from build123d import *

# Parameters (mm, degrees)
F0_W      = 42
F0_H      = 27
F1_DEPTH  = 3
F0_H_2    = 3
F2_DEPTH  = 45
F4_D      = 4
F6_D      = 5
F7_R      = 12
F8_DEPTH  = 25
F9_W      = 27
F9_H      = 3
F10_DEPTH = 4
F11_W     = 3
F11_H     = 4
F12_DEPTH = 25
F13_W     = 27
F13_H     = 3
F14_DEPTH = 4
F15_W     = 3
F15_H     = 4
F16_DEPTH = 25


with BuildPart() as f1:
    # F0 (on Top) → F1 (new body)
    with BuildSketch(Plane.XY):
        with Locations((0, 1.5)):
            Rectangle(F0_W, F0_H)
    extrude(amount=F1_DEPTH)

    # F0 (on Top) → F2 (join)
    with BuildSketch(Plane.XY):
        with Locations((0, -13.5)):
            Rectangle(F0_W, F0_H_2)
    extrude(amount=F2_DEPTH)

    # F4 (through all)
    with Locations(Plane.XY.offset(3)):
        with Locations((10, -8.5), (10, 11.5), (-10, 11.5), (-10, -8.5)):
            Hole(F4_D / 2)

    # F6 (through all)
    with Locations(Plane(origin=(0, -12, 0), x_dir=(-1, 0, 0), z_dir=(0, 1, 0))):
        with Locations((-15.5, 39.5), (-15.5, 8.5), (15.5, 8.5), (15.5, 39.5)):
            Hole(F6_D / 2)

    # F7 (on face) → F8 (cut)
    with BuildSketch(Plane(origin=(0, -12, 0), x_dir=(-1, 0, 0), z_dir=(0, 1, 0))):
        with Locations((0, 24)):
            Circle(F7_R)
    extrude(amount=-F8_DEPTH, mode=Mode.SUBTRACT)

    # F9 (on face) → F10 (join)
    with BuildSketch(Plane(origin=(-21, 0, 0), x_dir=(0, -1, 0), z_dir=(-1, 0, 0))):
        with Locations((-1.5, 1.5)):
            Rectangle(F9_W, F9_H)
    extrude(amount=F10_DEPTH)

    # F11 (on face) → F12 (cut)
    with BuildSketch(Plane.XY.offset(3)):
        with Locations((-23.5, 11)):
            Rectangle(F11_W, F11_H)
        with Locations((-23.5, -8)):
            Rectangle(F11_W, F11_H)
    extrude(amount=-F12_DEPTH, mode=Mode.SUBTRACT)

    # F13 (on face) → F14 (join)
    with BuildSketch(Plane.YZ.offset(21)):
        with Locations((1.5, 1.5)):
            Rectangle(F13_W, F13_H)
    extrude(amount=F14_DEPTH)

    # F15 (on face) → F16 (cut)
    with BuildSketch(Plane.XY.offset(3)):
        with Locations((23.5, 11)):
            Rectangle(F15_W, F15_H)
        with Locations((23.5, -8)):
            Rectangle(F15_W, F15_H)
    extrude(amount=-F16_DEPTH, mode=Mode.SUBTRACT)


solid = f1.part
Source: CAD feature listing. Evaluate the final solid. Frame: model axes, mm. A direction names the side the tool comes from. Round coordinates to 2 decimals unless told otherwise and drop trailing zeros. Loops run counter-clockwise (first coordinate to the right, second up) from the corner with the lowest first, then second, coordinate; pieces in that order, holes last. Notation, with made-up numbers: (81, 26.5) -> (87, 26.5) arc R25 cw to (87, 65.5) -> close; hole circle Ø10 at (-29, 63.5). An arc over 180 degrees is marked (long way). Answer as a JSON object with one key per item and string values. Group by question number.
Q1. Section query D-D (x = 0). Output: boundary loops of the cut face in (y, z).
Q2. Mould query, pull axis X, two halves, no side actions, for faces 6 (the flat face through (-25, -11, 2)), 7 (the flat face through (22, 11, 2)), 8 (the cylindrical face through (-17.5, -13.5, 7)), 9 (the flat face through (23, 13, 2)). Classes: pulls with the +X half, pulls with the -X half, needs draft (parallel to the pull), parting line crosses it, or undercut.
Q3. Ray query, line 1 (Z direction, x = -15.5, y = -12.8); line 2 (Y direction, x = 10, z = 2); line 3 (Z direction, x = 0, y = -13.25). Return the intervals inside material, ascending. Write a range as from..to.
Q4. Section query C-C (y = -8.5). Output: boundary loops of the cut face in (x, z).
Q5. Contact query for flat-ended pins moving along their axis: P1, Ø0.9, axis at x = 22, z = 2, coming from the -Y side; P2, Ø13.5, axis at x = -8, y = 7, coming from the +Z side; P3, Ø1.5, axis at x = -2, z = 36.5, coming from the +Y side. Output: stop coordinate, or through.
Q6. Section query A-A (z = 10). Output: boundary loops of the cut face in (x, y), plus the area to 3 significant figures.
Q7. Section query B-B (x = -15.5). Output: boundary loops of the cut face in (y, z), plus the area to 3 significant figures.
Q8. Access query for faces 1 (the flat face through (-24, 13, 2)), 2 (the flat face through (-23, -12, 1)), 3 (the flat face through (0, 0, 0)), 4 (the flat face through (0, 1, 3)), 5 (the flat face through (22, -8, 2)). Directions: +Z, -Z, +X, -X, +Y, -Y. A direction counts if a zero-diameter tool reaches every point of the face in a straight line with its end or side. Return the directions, or none.
Completed:
{
 "1": {"outline": "(-15, 0) -> (15, 0) -> (15, 3) -> (-12, 3) -> (-12, 12) -> (-15, 12) -> close; (-15, 36) -> (-12, 36) -> (-12, 45) -> (-15, 45) -> close"},
 "2": {"face 6": "pulls with the -X half", "face 7": "pulls with the +X half", "face 8": "undercut", "face 9": "needs draft"},
 "3": {"line 1": "0..6, 11..37, 42..45", "line 2": "-15..-10.5, -6.5..9.5, 13.5..15", "line 3": "0..12, 36..45"},
 "4": {"outline": "(-22, 0) -> (-12, 0) -> (-12, 3) -> (-22, 3) -> close; (-8, 0) -> (8, 0) -> (8, 3) -> (-8, 3) -> close; (12, 0) -> (22, 0) -> (22, 3) -> (12, 3) -> close"},
 "5": {"P1": "y = -12", "P2": "z = 3", "P3": "y = -12"},
 "6": {"outline": "(-21, -15) -> (-17.5, -15) -> (-17.5, -12) -> (-21, -12) -> close; (-13.5, -15) -> (13.5, -15) -> (13.5, -12) -> (-13.5, -12) -> close; (17.5, -15) -> (21, -15) -> (21, -12) -> (17.5, -12) -> close", "area": "102 mm²"},
 "7": {"outline": "(-15, 0) -> (15, 0) -> (15, 3) -> (-12, 3) -> (-12, 6) -> (-15, 6) -> close; (-15, 11) -> (-12, 11) -> (-12, 37) -> (-15, 37) -> close; (-15, 42) -> (-12, 42) -> (-12, 45) -> (-15, 45) -> close", "area": "186 mm²"},
 "8": {"face 1": "+Z, -Z, -X", "face 2": "+Z, -Z, -X, -Y", "face 3": "-Z, +X, -X, +Y, -Y", "face 4": "+Z, +X, -X, +Y", "face 5": "+Z, -Z, +X"}
}
